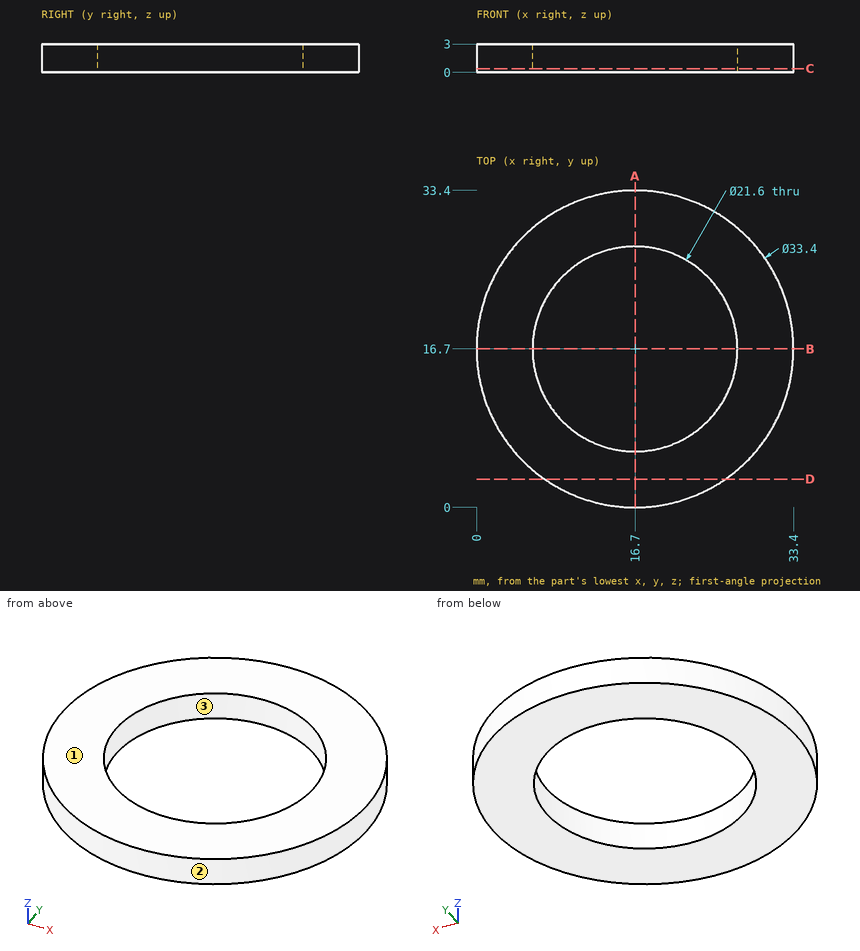
Verification items for this drawing (mm, ordinates from the low corner). Give positions to 0.01 mm unless a question says otherwise; leave off trailing zeros. Loops run counter-clockwise (first coordinate to the right, second up) from the corner with the lowest first, then second, coordinate; pieces in that order, holes last.
(1) Section check A-A on x = 16.7. Record the cut outline in (y, z).
From the geometry:
outline: (0, 0) - (5.9, 0) - (5.9, 3) - (0, 3) - close; (27.5, 0) - (33.4, 0) - (33.4, 3) - (27.5, 3) - close
(2) Thickness scan on L1, parallel to Y at x = 16.7, z = 1; L2, parallel to X at y = 21.5, z = 1.9; L3, parallel to Y at x = 8.5, z = 1.3. Record the ranges inside material, lowest first.
From the geometry:
L1: y = 0 to 5.9, 27.5 to 33.4
L2: x = 0.7 to 7.03, 26.37 to 32.7
L3: y = 2.15 to 9.67, 23.73 to 31.25
(3) Depth check by flat-ended pin: pin 1 Ø1.5 at (x, z) = (8.5, 1.5) entering from -Y. Enter the tip coordinate at first touch or a pass-through.
From the geometry:
pin 1: stops at y = 1.75
(4) Release check for a two-part mould opening along X. For the marked faces 1, 2 and 3 record: released by +X, released by -X, zero draft, split by the parting line, or undercut.
From the geometry:
face 1: zero draft
face 2: split by the parting line
face 3: undercut
(5) Section check D-D on y = 3. Record the cut outline in (x, z), then the cut area to 3 significant figures.
From the geometry:
outline: (7.15, 0) - (26.25, 0) - (26.25, 3) - (7.15, 3) - close
area: 57.3 mm2
(6) Section check C-C on z = 0.4. Record the cut outline in (x, y).
From the geometry:
outline: circle Ø33.4 at (16.7, 16.7); hole circle Ø21.6 at (16.7, 16.7)
